Autodesk Inventor part; units mm, degrees
ref_plane "Naeherungsschalter_Du8_XY" through (5, 0, 0) normal (0, 1, 0) x (1, 0, 0)
ref_plane "Naeherungsschalter_Du8_YZ" through (5, 0, 0) normal (1, 0, 0) x (0, 0, -1)
ref_plane "Naeherungsschalter_Du8_ZX" through (5, 0, 0) normal (0, 0, -1) x (0, 1, 0)
sketch "Skizze_1" plane through (0, 0, 0) normal (0, 1, 0) x (-1, 0, 0)
  line L0 (0, 10) -> (-4.5, 10)
  line L1 (-4.5, 10) -> (-4.5, 3.9686)
  arc A0 (-6, 3.873) -> (-4.5, 3.9686) centre (-5, 0) ccw
  line L2 (-6, 3.873) -> (-6, 10)
  line L3 (-6, 10) -> (-12, 10)
  line L4 (-12, 10) -> (-12, -10)
  line L5 (-12, -10) -> (0, -10)
  line L6 (0, -10) -> (0, 10)
extrude "Extrusion1" add sketch "Skizze_1" along normal blind 16
sketch "Sketch2" plane through (12, 0, 10) normal (1, 0, 0) x (0, 0, -1)
  point P0 (16.5, 4.25)
hole "Hole1" at (12, 4.25, -6.5) direction (-1, 0, 0) diameter 6 depth 3.2
sketch "Sketch3" plane through (12, 0, 10) normal (1, 0, 0) x (0, 0, -1)
  point P0 (16.5, 11.75)
hole "Hole2" at (12, 11.75, -6.5) direction (-1, 0, 0) diameter 6 depth 3.2
sketch "Skizze_5" plane through (8.8, 4.25, -6.5) normal (1, 0, 0) x (0, 0, -1)
  circle A0 centre (0, 0) radius 2.75
extrude "Extrusion2" add sketch "Skizze_5" along normal blind 3
sketch "Skizze_6" plane through (11.8, 4.25, -6.5) normal (1, 0, 0) x (0, 0, -1)
  line L0 (-1.25, -0.7217) -> (0, -1.4434)
  line L1 (0, -1.4434) -> (1.25, -0.7217)
  line L2 (1.25, -0.7217) -> (1.25, 0.7217)
  line L3 (1.25, 0.7217) -> (0, 1.4434)
  line L4 (0, 1.4434) -> (-1.25, 0.7217)
  line L5 (-1.25, 0.7217) -> (-1.25, -0.7217)
extrude "Extrusion3" cut sketch "Skizze_6" against normal blind 1.3
sketch "Skizze_4" plane through (8.8, 11.75, -6.5) normal (1, 0, 0) x (0, 0, -1)
  circle A0 centre (0, 0) radius 2.75
extrude "Extrusion4" add sketch "Skizze_4" along normal blind 3
sketch "Skizze_7" plane through (11.8, 11.75, -6.5) normal (1, 0, 0) x (0, 0, -1)
  line L0 (-1.25, -0.7217) -> (0, -1.4434)
  line L1 (0, -1.4434) -> (1.25, -0.7217)
  line L2 (1.25, -0.7217) -> (1.25, 0.7217)
  line L3 (1.25, 0.7217) -> (0, 1.4434)
  line L4 (0, 1.4434) -> (-1.25, 0.7217)
  line L5 (-1.25, 0.7217) -> (-1.25, -0.7217)
extrude "Extrusion5" cut sketch "Skizze_7" against normal blind 1.3
sketch "Sketch8" plane through (12, 0, 10) normal (1, 0, 0) x (0, 0, -1)
  point P0 (3.5, 8)
hole "Hole3" at (12, 8, 6.5) direction (-1, 0, 0) diameter 6 depth 3.2
sketch "Skizze_12" plane through (8.8, 8, 6.5) normal (1, 0, 0) x (0, 0, -1)
  circle A0 centre (0, 0) radius 2.75
extrude "Extrusion6" add sketch "Skizze_12" along normal blind 3
sketch "Skizze_13" plane through (11.8, 8, 6.5) normal (1, 0, 0) x (0, 0, -1)
  line L0 (-1.25, -0.7217) -> (0, -1.4434)
  line L1 (0, -1.4434) -> (1.25, -0.7217)
  line L2 (1.25, -0.7217) -> (1.25, 0.7217)
  line L3 (1.25, 0.7217) -> (0, 1.4434)
  line L4 (0, 1.4434) -> (-1.25, 0.7217)
  line L5 (-1.25, 0.7217) -> (-1.25, -0.7217)
extrude "Extrusion7" cut sketch "Skizze_13" against normal blind 1.3
ref_plane "Naeherungsschalter_Du8_XY" through (5, 0, 0) normal (0, 1, 0) x (1, 0, 0)
ref_plane "Naeherungsschalter_Du8_YZ" through (5, 0, 0) normal (1, 0, 0) x (0, 0, -1)
ref_plane "Naeherungsschalter_Du8_ZX" through (5, 0, 0) normal (0, 0, -1) x (0, 1, 0)
ref_plane "apzbplus_XY" through (4.5, 11.75, -6.5) normal (0, 1, 0) x (1, 0, 0)
ref_plane "apzbplus_YZ" through (4.5, 11.75, -6.5) normal (1, 0, 0) x (0, 0, -1)
ref_plane "apzbplus_ZX" through (4.5, 11.75, -6.5) normal (0, 0, -1) x (0, 1, 0)
ref_plane "jgz64_XY" through (0, 8, 6.5) normal (0, 0, 1) x (1, 0, 0)
ref_plane "jgz64_YZ" through (0, 8, 6.5) normal (1, 0, 0) x (0, 1, 0)
ref_plane "jgz64_ZX" through (0, 8, 6.5) normal (0, 1, 0) x (0, 0, 1)
ref_plane "jpg64_XY" through (0, 11, 0) normal (1, 0, 0) x (0, 0, -1)
ref_plane "jpg64_YZ" through (0, 11, 0) normal (0, 0, -1) x (0, 1, 0)
ref_plane "jpg64_ZX" through (0, 11, 0) normal (0, 1, 0) x (1, 0, 0)
ref_plane "klh1_XY" through (0, 11.75, -6.5) normal (1, 0, 0) x (0, 0, -1)
ref_plane "klh1_YZ" through (0, 11.75, -6.5) normal (0, 0, -1) x (0, 1, 0)
ref_plane "klh1_ZX" through (0, 11.75, -6.5) normal (0, 1, 0) x (1, 0, 0)
ref_plane "klh_64_XY" through (0, 8, -6.5) normal (1, 0, 0) x (0, 0, -1)
ref_plane "klh_64_YZ" through (0, 8, -6.5) normal (0, 0, -1) x (0, 1, 0)
ref_plane "klh_64_ZX" through (0, 8, -6.5) normal (0, 1, 0) x (1, 0, 0)
ref_plane "klh_80_XY" through (0, 4.25, -6.5) normal (1, 0, 0) x (0, 0, -1)
ref_plane "klh_80_YZ" through (0, 4.25, -6.5) normal (0, 0, -1) x (0, 1, 0)
ref_plane "klh_80_ZX" through (0, 4.25, -6.5) normal (0, 1, 0) x (1, 0, 0)
ref_plane "pzn_300_380_XY" through (4.5, 8, 6.5) normal (0, 0, 1) x (1, 0, 0)
ref_plane "pzn_300_380_YZ" through (4.5, 8, 6.5) normal (1, 0, 0) x (0, 1, 0)
ref_plane "pzn_300_380_ZX" through (4.5, 8, 6.5) normal (0, 1, 0) x (0, 0, 1)
ref_plane "vst___geh_XY" through (0, 0, 0) normal (1, 0, 0) x (0, 0, -1)
ref_plane "vst___geh_YZ" through (0, 0, 0) normal (0, 0, -1) x (0, 1, 0)
ref_plane "vst___geh_ZX" through (0, 0, 0) normal (0, 1, 0) x (1, 0, 0)
ref_plane "vst___geh_2_XY" through (0, 16, 0) normal (1, 0, 0) x (0, 0, -1)
ref_plane "vst___geh_2_YZ" through (0, 16, 0) normal (0, 0, -1) x (0, 1, 0)
ref_plane "vst___geh_2_ZX" through (0, 16, 0) normal (0, 1, 0) x (1, 0, 0)
properties part number "SCHUNK-5503506 Halter fuer NHS KL03"
CAD build for the part. Positions are in the model's coordinates, mm. A direction names the side the tool comes from. Give positions to 0.01 mm unless a question says otherwise; leave off trailing zeros. Order: outer loops, then holes, each group sorted by start corner. A loop starts at its lowest first (then second) coordinate and runs counter-clockwise, first axis right, second up. Notation, with made-up numbers: M 17,80.25 L 58,80.25 A23 cw 58,97.25 Z; hole C -5.75,-25 d1. An arc over 180 degrees is marked long. Put each result on its own line as item: value. Start each with the question number.
(1) Which spindle directions (+Z, -Z, +X, -X, +Y, -Y) get a long thin tool onto all of the face, cutting with end or side? Do faces 4 (the flat face through (12, 8, 0)), 5 (the flat face through (11.159, 3.162, -7.116)). Say none if no direction does.
(2) Flat gauge pins, fed straight in: pin 1 Ø3 at (y, z) = (4, -6) entering from +X; pin 2 Ø0.8 at (y, z) = (4, -7) entering from +X. Where does each tip first touch, or does it go through?
(3) Saw through at A-A, the plane y = 4.25. Write the cut outline in (x, z), then the cut area to 3 significant figures.
(4) Drill centre lines: line 1 along Y through (x, z) = (10.2, 6.5); line 2 along Y through (x, z) = (10.35, -6.5); line 3 along X through (y, z) = (7.75, 8.5). Where is each one in solid material? Low to high.
(5) Saw through at C-C, the plane z = 8.5. Write the cut outline in (x, y), then the cut area to 3 significant figures.
(6) Saw through at D-D, the plane x = 5. Write the cut outline in (y, z).
(7) Mould opens along Z. For faces 1 (the flat face through (9, 8, 10)), 2 (the flat face through (9, 16, -2)), 3 (the flat face through (11.16, 6.92, 7.13)) say: +Z half, -Z half, draft (parallel to the pull), parting line (faces both ways), or undercut.
(8) Saw through at B-B, the plane x = 1.5. Write the cut outline in (y, z).
Check result:
1. face 4: +Z, -Z, +X, +Y, -Y
1. face 5: +X
2. pin 1: stops at x = 11.8
2. pin 2: stops at x = 10.5
3. outline: M 0,-10 L 12,-10 L 12,-9.5 L 8.8,-9.5 L 8.8,-9.25 L 11.8,-9.25 L 11.8,-7.75 L 10.5,-7.75 L 10.5,-5.25 L 11.8,-5.25 L 11.8,-3.75 L 8.8,-3.75 L 8.8,-3.5 L 12,-3.5 L 12,10 L 6,10 L 6,3.87 A4 cw long 4.5,3.97 L 4.5,10 L 0,10 Z
3. area: 175 mm2
4. line 1: y = 0 to 5, 5.25 to 10.75, 11 to 16
4. line 2: y = 0 to 1.25, 1.5 to 7, 7.25 to 8.75, 9 to 14.5, 14.75 to 16
4. line 3: x = 0 to 4.5, 6 to 11.8
5. outline: M 0,0 L 4.5,0 L 4.5,16 L 0,16 Z; M 6,0 L 12,0 L 12,5.76 L 8.8,5.76 L 8.8,6.11 L 11.8,6.11 L 11.8,9.89 L 8.8,9.89 L 8.8,10.24 L 12,10.24 L 12,16 L 6,16 Z
5. area: 165 mm2
6. outline: M 0,-10 L 16,-10 L 16,-4 L 0,-4 Z
7. face 1: +Z half
7. face 2: draft
7. face 3: undercut
8. outline: M 0,-10 L 16,-10 L 16,-1.94 L 0,-1.94 Z; M 0,1.94 L 16,1.94 L 16,10 L 0,10 Z
